Answer from the drawing. Dimensions are ordinates in mm from the lowest x, y and z of the part. Round coordinates to 2 decimals unless told otherwise and drop trailing zeros. Write each loop counter-clockwise with the first axis right and the second up, starting at its lowest first coordinate (ties: lowest second). Pieces come first, ordered by that corner, then holes. Notation, with made-up numbers: (-26.75, 23.5) - (7.25, 23.5) arc R26 cw to (7.25, 53.5) - close; hole circle Ø10 at (35, -20). An arc over 180 degrees is marked (long way). Answer in a Markdown table with one row per item.
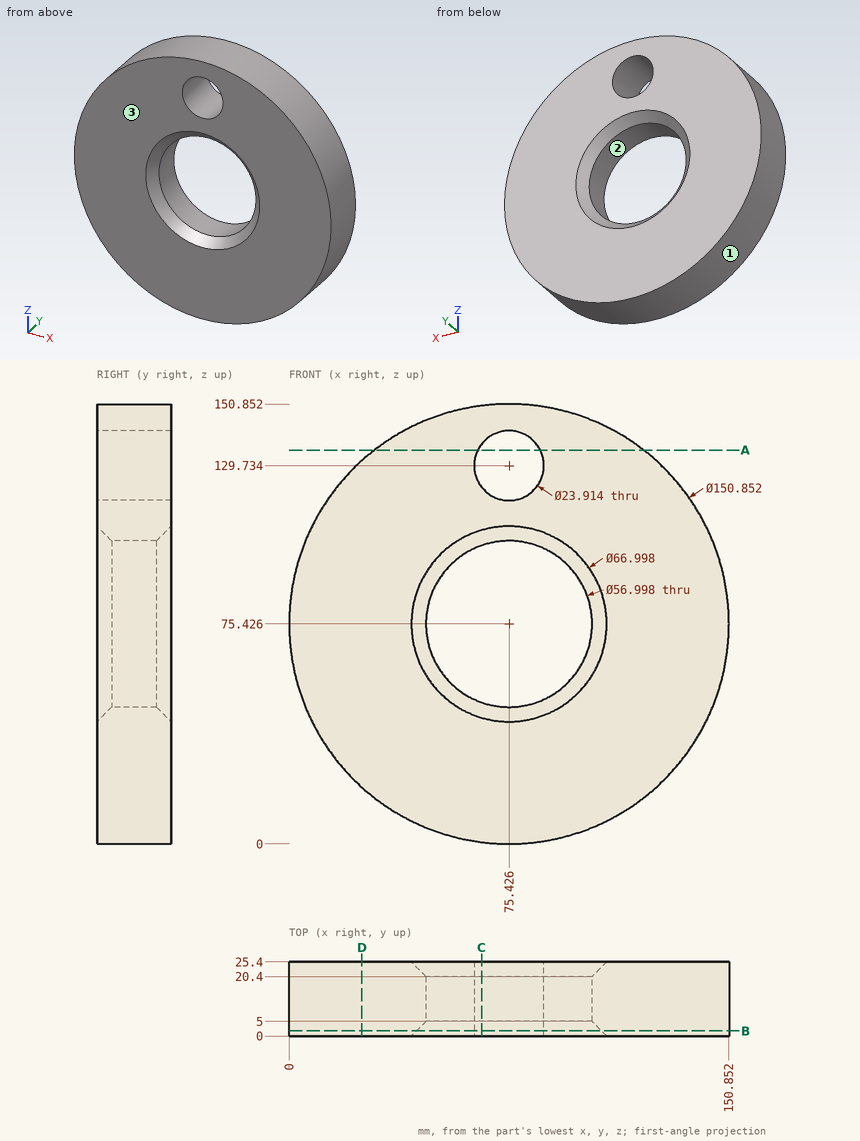
(1) Section B-B (y = 1.75) is taken. Give the vertices of the cut face in (x, z) (1 decimal).
Checked values:
| item | result |
|---|---|
| outline | circle Ø150.9 at (75.4, 75.4); hole circle Ø63.5 at (75.4, 75.4); hole circle Ø23.9 at (75.4, 129.7) |
(2) Section A-A (z = 135) is taken. Give the vertices of the cut face in (x, y) (1 decimal), and give its area (3 significant figures).
Checked values:
| item | result |
|---|---|
| outline | (29.2, 0) - (64.7, 0) - (64.7, 25.4) - (29.2, 25.4) - close; (86.2, 0) - (121.7, 0) - (121.7, 25.4) - (86.2, 25.4) - close |
| area | 1,800 mm2 |
(3) Section C-C (x = 66) is taken. State how many separate pieces and enclosed holes the cut face has, and give its area (3 significant figures).
Checked values:
| item | result |
|---|---|
| separate pieces | 3 |
| enclosed holes | 0 |
| area | 2,010 mm2 |
(4) Section D-D (x = 25) is taken. Give the vertices of the cut face in (y, z), and give its area (3 significant figures).
Checked values:
| item | result |
|---|---|
| outline | (0, 19.33) - (25.4, 19.33) - (25.4, 131.52) - (0, 131.52) - close |
| area | 2,850 mm2 |
(5) Flat-ended cylindrical pins translate along their axes: pin 1 (12 mm diameter, centred on x = 26.5, y = 22, fed in from -Z); pin 2 (2 mm diameter, centred on x = 133.5, z = 33, fed in from -Y); pin 3 (12 mm diameter, centred on x = 89.5, y = 12, fed in from -Z); pin 4 (2 mm diameter, centred on y = 7.5, z = 68.5, fed in from +X). Find the tip coordinate at first contact, or state that the pin passes through.
Checked values:
| item | result |
|---|---|
| pin 1 | stops at z = 13.41 |
| pin 2 | stops at y = 0 |
| pin 3 | stops at z = 0.43 |
| pin 4 | stops at x = 150.62 |
(6) Find the intervals of material crossed by line 1 (X direction, y = 19.75, z = 67); line 2 (X direction, y = 21.5, z = 75); line 3 (Z direction, x = 71, y = 14.25), in increasing order.
Checked values:
| item | result |
|---|---|
| line 1 | x = 0.47 to 48.2, 102.65 to 150.38 |
| line 2 | x = 0 to 45.83, 105.02 to 150.85 |
| line 3 | z = 0.13 to 47.27, 103.58 to 118.63, 140.84 to 150.72 |
(7) For a pull along Z with two mould halves and no side action, classify the marked faces 1, 2 and 3 as pulls with the +Z half, pulls with the -Z half, needs draft (parallel to the pull), parting line crosses it, or undercut.
Checked values:
| item | result |
|---|---|
| face 1 | parting line crosses it |
| face 2 | undercut |
| face 3 | needs draft |
